The model under review builds one solid part; all positions refer to its coordinate system, in mm. A direction names the side the tool comes from. Coordinates: 2 decimals unless noted, no trailing zeros. Write each loop counter-clockwise with the first axis right and the second up, starting at its lowest first coordinate (ties: lowest second). Pieces come first, ordered by that corner, then holes. Notation, with made-up numbers: (16.25, 32) -> (40.25, 32) arc R19 ccw to (40.25, 53) -> close; hole circle Ø2 at (-18, 84.25). An arc over 180 degrees is marked (long way). Write each question's results on one line, items separated by ' | '.
```python
from build123d import *

# Parameters (mm, degrees)
SKETCH1_W           = 50.8
SKETCH1_H           = 127
SKETCH1_R           = 3.96875
SKETCH1_R_2         = 3.3734375
BOSS_EXTRUDE2_DEPTH = 6.985


with BuildPart() as part:
    # Sketch1 → Boss-Extrude2 (new body)
    with BuildSketch(Plane.XY):
        with Locations((25.4, 63.5)):
            Rectangle(SKETCH1_W, SKETCH1_H)
        with Locations((25.4, 12.7)):
            Circle(SKETCH1_R, mode=Mode.SUBTRACT)
        with Locations((25.4, 116.84)):
            Circle(SKETCH1_R_2, mode=Mode.SUBTRACT)
        with Locations((25.4, 91.44)):
            Circle(SKETCH1_R_2, mode=Mode.SUBTRACT)
        with BuildLine():
            ThreePointArc((42.2275, 51.256646253), (25.4, 54.76875), (8.5725, 51.256646253))
            ThreePointArc((8.5725, 51.256646253), (6.522580542, 46.031726796), (11.7475, 43.981807338))
            ThreePointArc((11.7475, 43.981807338), (25.4, 46.83125), (39.0525, 43.981807338))
            ThreePointArc((39.0525, 43.981807338), (44.277419458, 46.031726796), (42.2275, 51.256646253))
        make_face(mode=Mode.SUBTRACT)
    extrude(amount=BOSS_EXTRUDE2_DEPTH)


solid = part.part
```
Q1. Add section B-B (z = 4.75). Write out the cut boundary in (x, y).
Solution:
outline: (0, 0) -> (50.8, 0) -> (50.8, 127) -> (0, 127) -> close; hole (8.57, 51.26) arc R3.97 ccw to (11.75, 43.98) arc R34.13 cw to (39.05, 43.98) arc R3.97 ccw to (42.23, 51.26) arc R42.07 ccw to start; hole circle Ø7.94 at (25.4, 12.7); hole circle Ø6.75 at (25.4, 91.44); hole circle Ø6.75 at (25.4, 116.84)
Q2. Add section D-D (x = 31). Write out the cut boundary in (y, z) (3 decimals), plus the area to 3 significant figures.
Solution:
outline: (0, 0) -> (46.369, 0) -> (46.369, 6.985) -> (0, 6.985) -> close; (54.394, 0) -> (127, 0) -> (127, 6.985) -> (54.394, 6.985) -> close | area: 831 mm²
Q3. For line 1 (Y direction, x = 25, z = 3.75); line 2 (Y direction, x = 27, z = 4); line 3 (Y direction, x = 9, z = 6.25), list the stretches that pass through material, from the lowest coordinate up. Write a range as from..to.
Solution:
line 1: 0..8.75, 16.65..46.83, 54.77..88.09, 94.79..113.49, 120.19..127 | line 2: 0..9.07, 16.33..46.79, 54.74..88.47, 94.41..113.87, 119.81..127 | line 3: 0..43.82, 51.44..127
Q4. Machinability: for faces 1 (the cylindrical face through (25.64, 54.77, 3.44)), 2 (the flat face through (25, 0, 3)), which of the approach directions +Z, -Z, +X, -X, +Y, -Y give a long, thin tool a straight path to every point of the face, cutting with its end or side? Answer none if there is none.
Solution:
face 1: +Z, -Z | face 2: +Z, -Z, +X, -X, -Y
Q5. Draft analysis for pull direction X (two halves, no side actions). For faces 3 (the flat face through (50.8, 63, 3)), 4 (the cylindrical face through (25.2, 46.83, 3.44)), 5 (the flat face through (0, 63, 3)), state which applies: pulls with the +X half, pulls with the -X half, needs draft (parallel to the pull), parting line crosses it, or undercut.
Solution:
face 3: pulls with the +X half | face 4: undercut | face 5: pulls with the -X half
Q6. Add section C-C (x = 25.4). Write out the cut boundary in (y, z) (3 decimals), plus the area to 3 significant figures.
Solution:
outline: (0, 0) -> (8.731, 0) -> (8.731, 6.985) -> (0, 6.985) -> close; (16.669, 0) -> (46.831, 0) -> (46.831, 6.985) -> (16.669, 6.985) -> close; (54.769, 0) -> (88.067, 0) -> (88.067, 6.985) -> (54.769, 6.985) -> close; (94.813, 0) -> (113.467, 0) -> (113.467, 6.985) -> (94.813, 6.985) -> close; (120.213, 0) -> (127, 0) -> (127, 6.985) -> (120.213, 6.985) -> close | area: 682 mm²
Q7. Add section A-A (y = 91.44). Write out the cut boundary in (x, z) (3 decimals), plus the area to 3 significant figures.
Solution:
outline: (0, 0) -> (22.027, 0) -> (22.027, 6.985) -> (0, 6.985) -> close; (28.773, 0) -> (50.8, 0) -> (50.8, 6.985) -> (28.773, 6.985) -> close | area: 308 mm²
